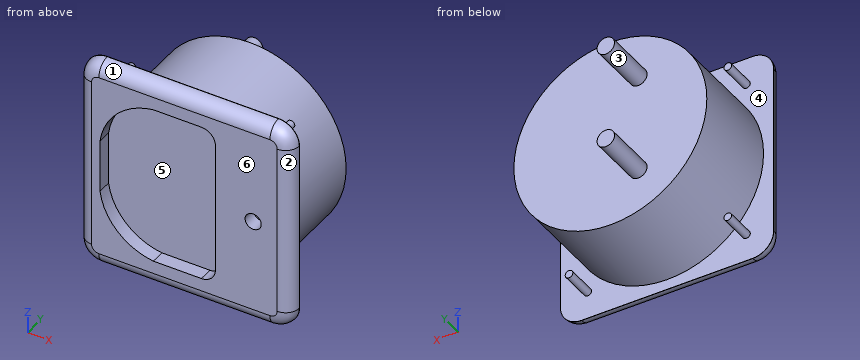
Autodesk Inventor part; units mm, degrees
ref_plane "YZ Plane" through (0, 0, 0) normal (1, 0, 0) x (0, 1, 0)
ref_plane "XZ Plane" through (0, 0, 0) normal (0, 1, 0) x (-1, 0, 0)
ref_plane "XY Plane" through (0, 0, 0) normal (0, 0, 1) x (1, 0, 0)
sketch "Sketch1" plane through (0, 0, 0) normal (0, 1, 0) x (-1, 0, 0)
  line L0 (-38.095, 38.17) -> (38.095, 38.17)
  line L1 (38.095, 38.17) -> (38.095, -38.17)
  line L2 (38.095, -38.17) -> (-38.095, -38.17)
  line L3 (-38.095, -38.17) -> (-38.095, 38.17)
  line L4 (-38.095, 38.17) -> (38.095, -38.17) construction
  line L5 (38.095, 38.17) -> (-38.095, -38.17) construction
  line L6 (-6.095, 28.615) -> (11.095, 28.615)
  line L7 (11.095, -28.615) -> (-6.095, -28.615)
  line L8 (-11.095, -23.615) -> (-11.095, 23.615)
  line L9 (-11.095, 28.615) -> (11.095, -28.615) construction
  line L10 (11.095, 28.615) -> (-11.095, -28.615) construction
  line L11 (30.1625, 9.5) -> (30.1625, -9.5)
  arc A0 (30.1625, 9.5) -> (11.095, 28.615) centre (8.2631, 6.7226) ccw
  line L12 (38.095, 0) -> (-38.095, 0)
  arc A1 (11.095, -28.615) -> (30.1625, -9.5) centre (8.2631, -6.7226) ccw
  arc A2 (-6.095, 28.615) -> (-11.095, 23.615) centre (-6.095, 23.615) ccw
  arc A3 (-11.095, -23.615) -> (-6.095, -28.615) centre (-6.095, -23.615) ccw
  line L13 (-11.095, 0) -> (-38.095, 0)
  circle A4 centre (-24.595, 0) radius 2.89
  point P0 (0, 0)
  dimension "d0" = 76.34
  dimension "d1" = 76.19
  dimension "d2" = 57.23
  dimension "d3" = 22.19
  dimension "d5" = 5
  dimension "d6" = 5
  dimension "d7" = 5.78
extrude "Extrusion1" add sketch "Sketch1" along normal blind 5 contours L0 L1 L12 L11 A0 L6 A2 L8 A4 L3 | L12 A4 L8 A3 L7 A1 L11 L1 L2 L3
sketch "Sketch2" plane through (0, 5, 0) normal (0, 1, 0) x (1, 0, 0)
  circle A0 centre (0, 0) radius 34.5
  dimension "d10" = 69
extrude "Extrusion2" add sketch "Sketch2" along normal blind 33.12
sketch "Sketch3" plane through (0, 5, 0) normal (0, 1, 0) x (1, 0, 0)
  line L0 (28.385, 28.385) -> (-28.385, 28.385)
  line L1 (-28.385, 28.385) -> (-28.385, -28.385)
  line L2 (-28.385, -28.385) -> (28.385, -28.385)
  line L3 (28.385, -28.385) -> (28.385, 28.385)
  line L4 (28.385, 28.385) -> (-28.385, -28.385) construction
  line L5 (-28.385, 28.385) -> (28.385, -28.385) construction
  circle A0 centre (28.385, -28.385) radius 1.375
  circle A1 centre (-28.385, 28.385) radius 1.375
  circle A2 centre (-28.385, -28.385) radius 1.375
  circle A3 centre (28.385, 28.385) radius 1.375
  point P0 (0, 0)
  dimension "d13" = 56.77
  dimension "d14" = 56.77
  dimension "d15" = 2.75
  dimension "d16" = 2.75
  dimension "d18" = 2.75
  dimension "d19" = 2.75
extrude "Extrusion3" add sketch "Sketch3" along normal blind 10.9 contours A1 L1 L0 | L0 L1 A1 | A3 L3 L0 | L0 L3 A3 | A2 L2 L1 | L1 L2 A2 | A0 L2 L3 | L3 L2 A0
sketch "Sketch5" plane through (0, 38.12, 0) normal (0, 1, 0) x (1, 0, 0)
  line L0 (10, 17.5) -> (-10, 17.5)
  line L1 (-10, 17.5) -> (-10, -17.5)
  line L2 (-10, -17.5) -> (10, -17.5)
  line L3 (10, -17.5) -> (10, 17.5)
  line L4 (10, 17.5) -> (-10, -17.5) construction
  line L5 (-10, 17.5) -> (10, -17.5) construction
  circle A0 centre (-10, 17.5) radius 3.125
  circle A1 centre (-10, -17.5) radius 3.125
  point P0 (0, 0)
  dimension "d32" = 35
  dimension "d33" = 20
  dimension "d34" = 6.25
  dimension "d35" = 6.25
extrude "Extrusion5" add sketch "Sketch5" along normal blind 19 contours A0 L1 L0 | L0 L1 A0 | A1 L1 L2 | L2 L1 A1
fillet "Fillet1" radius 7.5 4 edges at (-38.095, 2.5, 38.17) (38.095, 2.5, 38.17) (38.095, 2.5, -38.17) (-38.095, 2.5, -38.17)
fillet "Fillet2" radius 4.9 8 edges at (-35.8983, 0, -35.9733) (-38.095, 0, 0) (-35.8983, 0, 35.9733) (0, 0, 38.17) (35.8983, 0, 35.9733) (38.095, 0, 0) (35.8983, 0, -35.9733) (0, 0, -38.17)
properties part number "MarionEICdcAmeter" material "Acetal Resin, Black"
Design review of the part built by this model. Coordinates are the model's own, in mm. Face numbers are marked on the shaded views. A direction names the side the tool comes from. Give positions to 0.01 mm unless a question says otherwise; leave off trailing zeros. Loops run counter-clockwise (first coordinate to the right, second up) from the corner with the lowest first, then second, coordinate; pieces in that order, holes last. Notation, with made-up numbers: (-3.75, -22) -> (33.25, -22) arc R13 ccw to (33.25, -2) -> close; hole circle Ø8 at (35, 23). An arc over 180 degrees is marked (long way). Write each question's results on one line, items separated by ' | '.
Q1. Take a section at C-C, the plane y = 45.5. Write out the cut boundary in (x, z) (3 decimals).
Reply:
outline: circle Ø6.25 at (-10, -17.5); circle Ø6.25 at (-10, 17.5)
Q2. Take a section at D-D, the plane x = 0. Write out the cut boundary in (y, z) (3 decimals), plus the area to 3 significant figures.
Reply:
outline: (0, -33.27) arc R4.9 ccw to (4.9, -38.17) -> (5, -38.17) -> (5, -34.5) -> (38.12, -34.5) -> (38.12, 34.5) -> (5, 34.5) -> (5, 38.17) -> (4.9, 38.17) arc R4.9 ccw to (0, 33.27) -> (0, 28.615) -> (5, 28.615) -> (5, -28.615) -> (0, -28.615) -> close | area: 2,370 mm²
Q3. Wall thickness on L1, parallel to X at y = 1.4, z = 0 (1 decimal); L2, parallel to X at y = 2.3, z = 0 (1 decimal); L3, parallel to Y at x = -3.5, z = 11: over which ranges is each line inside the solid? List them lowest first.
Reply:
L1: x = -36.6 to -30.2, 11.1 to 21.7, 27.5 to 36.6 | L2: x = -37.3 to -30.2, 11.1 to 21.7, 27.5 to 37.3 | L3: y = 5 to 38.12
Q4. The part is to be moulded in two halves that separate along Z. For the marked faces 1, 2 and 3, say which applies: +Z half, -Z half, draft (parallel to the pull), parting line (faces both ways), or undercut.
Reply:
face 1: +Z half | face 2: draft | face 3: undercut
Q5. Take a section at A-A, the plane y = 10. Write out the cut boundary in (x, z) (3 decimals), plus the area to 3 significant figures.
Reply:
outline: circle Ø69 at (0, 0); circle Ø2.75 at (-28.385, -28.385); circle Ø2.75 at (-28.385, 28.385); circle Ø2.75 at (28.385, -28.385); circle Ø2.75 at (28.385, 28.385) | area: 3,760 mm²
Q6. For pin 1 Ø2 at (x, z) = (28, 28.5) entering from +Y; pin 2 Ø12 at (y, z) = (36, 14.5) entering from +X; pin 3 Ø1.5 at (x, y) = (7, 37.5) entering from +Z, all flat-tipped, find the tip position at first contact; note any pin that passes through.
Reply:
pin 1: stops at y = 15.9 | pin 2: stops at x = 33.44 | pin 3: stops at z = 33.93
Q7. Machinability: for the marked faces 4, 5 and 6, which of the approach directions +Z, -Z, +X, -X, +Y, -Y give a long, thin tool a straight path to every point of the face, cutting with its end or side? Answer none if there is none.
Reply:
face 4: +Y | face 5: -Y | face 6: +Z, -Z, +X, -X, -Y
